Geometry: see drawing. Coordinates: mm, zero at the bounding-box minimum. A direction names the side the tool comes from. Round coordinates to 2 decimals unless told otherwise and drop trailing zeros. Order: outer loops, then holes, each group sorted by start corner. A loop starts at its lowest first (then second) coordinate and runs counter-clockwise, first axis right, second up. Notation, with made-up numbers: (-12.75, 74.25) -> (33.25, 74.25) arc R7 cw to (33.25, 78.25) -> close; hole circle Ø7 at (8, 56.25). An arc over 180 degrees is marked (long way). Use a Markdown table: item, result.
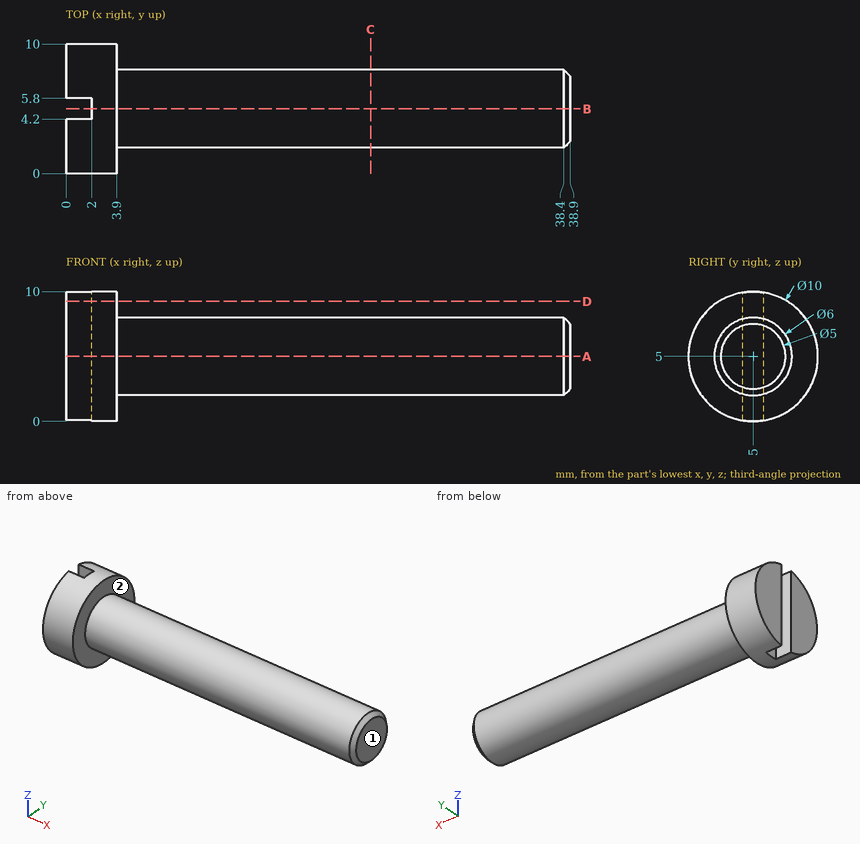
1) Set-up query: the marked faces 1 and 2. Return all of +Z, -Z, +X, -X, +Y, -Y with unobstructed straight access to the full face (end or side cutting, diameter ignored); none if empty.
Answer key:
| item | result |
|---|---|
| face 1 | +Z, -Z, +X, +Y, -Y |
| face 2 | +X |
2) Contact query for flat-ended pins moving along their axis: P1, Ø1, axis at x = 1, z = 6.5, coming from the +Y side; P2, Ø5, axis at x = 28.5, y = 1.5, coming from the -Z side; P3, Ø1.3, axis at y = 5, z = 3, coming from the -X side. Output: stop coordinate, or through.
Answer key:
| item | result |
|---|---|
| P1 | stops at y = 9.9 |
| P2 | stops at z = 2.17 |
| P3 | stops at x = 2 |
3) Ray query, probe 1 along X at (y, z) = (7.5, 7.5); probe 2 along X at (y, z) = (5, 1.5); probe 3 along Z at (x, y) = (11, 2.5). Return the intervals inside material, ascending.
Answer key:
| item | result |
|---|---|
| probe 1 | x = 0 to 3.9 |
| probe 2 | x = 2 to 3.9 |
| probe 3 | z = 3.34 to 6.66 |
4) Cut plane A-A on z = 5. Return loops of the section in (x, y), and give its area (3 significant figures).
Answer key:
| item | result |
|---|---|
| outline | (0, 0) -> (3.9, 0) -> (3.9, 2) -> (38.4, 2) -> (38.9, 2.5) -> (38.9, 7.5) -> (38.4, 8) -> (3.9, 8) -> (3.9, 10) -> (0, 10) -> (0, 5.8) -> (2, 5.8) -> (2, 4.2) -> (0, 4.2) -> close |
| area | 246 mm^2 |
5) Cut plane B-B on y = 5. Return loops of the section in (x, z), and give its area (3 significant figures).
Answer key:
| item | result |
|---|---|
| outline | (2, 0) -> (3.9, 0) -> (3.9, 2) -> (38.4, 2) -> (38.9, 2.5) -> (38.9, 7.5) -> (38.4, 8) -> (3.9, 8) -> (3.9, 10) -> (2, 10) -> close |
| area | 229 mm^2 |
6) Cut plane C-C on x = 23.5. Return loops of the section in (y, z).
Answer key:
| item | result |
|---|---|
| outline | circle Ø6 at (5, 5) |
7) Cut plane D-D on z = 9.25. Return loops of the section in (x, y), and give its area (3 significant figures).
Answer key:
| item | result |
|---|---|
| outline | (0, 2.37) -> (3.9, 2.37) -> (3.9, 7.63) -> (0, 7.63) -> (0, 5.8) -> (2, 5.8) -> (2, 4.2) -> (0, 4.2) -> close |
| area | 17.3 mm^2 |
